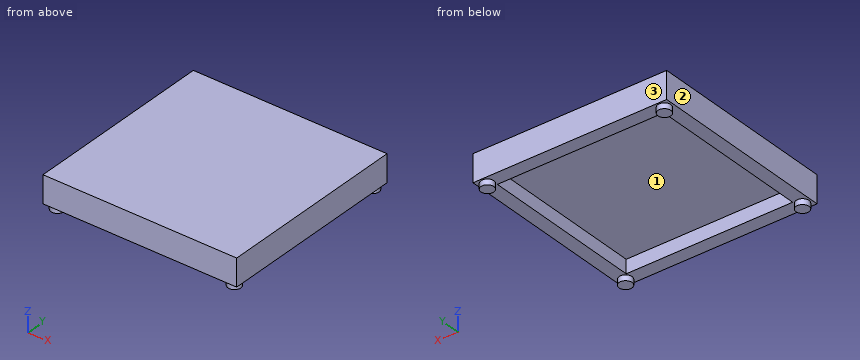
```python
from build123d import *

# Parameters (mm, degrees)
F0_W     = 71
F0_H     = 70
F1_DEPTH = 10
F2_T     = -5
F3_R     = 2.36344
F4_R     = 2.36344
F7_DEPTH = 2
F5_R     = 2.36344
F6_R     = 2.36344
F8_DEPTH = 2


with BuildPart() as f1:
    # F0 (on Top) → F1 (new body)
    with BuildSketch(Plane.XY):
        Rectangle(F0_W, F0_H)
    extrude(amount=F1_DEPTH)

    # F2
    f2_openings = [f1.faces().sort_by_distance(p)[0] for p in [
        (0, 0, 0),
    ]]
    offset(amount=F2_T, openings=f2_openings)

    # F3 (on face) + F4 (on Top) → F7 (join)
    with BuildSketch(Plane(origin=(0, 0, 0), x_dir=(1, 0, 0), z_dir=(0, 0, -1))):
        with Locations((-32.44344, 32.1634384014)):
            Circle(F3_R)
    with BuildSketch(Plane.XY):
        with Locations((32.44344, -32.1634384014)):
            Circle(F4_R)
    extrude(amount=F7_DEPTH, dir=(0, 0, -1))

    # F5 (on face) + F6 (on face) → F8 (join)
    with BuildSketch(Plane(origin=(0, 0, 0), x_dir=(1, 0, 0), z_dir=(0, 0, -1))):
        with Locations((-32.44344, -32.1634384014)):
            Circle(F5_R)
    with BuildSketch(Plane(origin=(0, 0, 0), x_dir=(1, 0, 0), z_dir=(0, 0, -1))):
        with Locations((32.44344, -32.1634384014)):
            Circle(F6_R)
    extrude(amount=F8_DEPTH)


solid = f1.part
```
CAD build for the part. Positions are in the model's coordinates, mm. Face numbers are marked on the shaded views. Round coordinates to 2 decimals unless told otherwise and drop trailing zeros. Order: outer loops, then holes, each group sorted by start corner. A loop starts at its lowest first (then second) coordinate and runs counter-clockwise, first axis right, second up.
Q1. Slice it at B-B (z = 2). Write the cut outline in (x, y), and give its area (3 significant figures).
Q2. Slice it at A-A (x = 23). Write the cut outline in (y, z), and give its area (3 significant figures).
Q3. Drop a flat-ended pin along its axis: pin 1 (21 mm diameter, centred on x = -2, y = -6, fed in from -Z). Give the stop position or say it passes through.
Q4. Slice it at C-C (y = -14). Write the cut outline in (x, z), and give its area (3 significant figures).
Q5. Wall check: L1, parallel to X at y = 4, z = 4.75; L2, parallel to Y at x = 29.5, z = 2; L3, parallel to Z at x = 10, y = 3. Give the ranges that are in metal, low to high.
Q6. Two-plate mould, pull along X, no slides. Class the marked faces 1, 2 and 3: pulls with the +X half, pulls with the -X half, needs draft (parallel to the pull), parting line crosses it, or undercut.
Results below:
1. outline: (-35.5, -35) - (35.5, -35) - (35.5, 35) - (-35.5, 35) - close; hole (-30.5, -30) - (30.5, -30) - (30.5, 30) - (-30.5, 30) - close
1. area: 1,310 mm2
2. outline: (-35, 0) - (-30, 0) - (-30, 5) - (30, 5) - (30, 0) - (35, 0) - (35, 10) - (-35, 10) - close
2. area: 400 mm2
3. pin 1: stops at z = 5
4. outline: (-35.5, 0) - (-30.5, 0) - (-30.5, 5) - (30.5, 5) - (30.5, 0) - (35.5, 0) - (35.5, 10) - (-35.5, 10) - close
4. area: 405 mm2
5. L1: x = -35.5 to -30.5, 30.5 to 35.5
5. L2: y = -35 to -30, 30 to 35
5. L3: z = 5 to 10
6. face 1: undercut
6. face 2: pulls with the -X half
6. face 3: needs draft
